Source: three-view drawing plus pictorial views. Frame: mm from the lowest corner of the part. A direction names the side the tool comes from. Give positions to 0.01 mm unless a question says otherwise; leave off trailing zeros. Write each loop counter-clockwise with the first axis right and the second up, starting at its lowest first coordinate (ties: lowest second). Pieces come first, ordered by that corner, then holes. Notation, with made-up numbers: (1, 17) -> (39, 17) arc R16 cw to (39, 47) -> close; hole circle Ø7 at (15.25, 10.5). An arc over 180 degrees is marked (long way). Answer in a Markdown table with one row per item. Add a question column.
Item 1: First-contact query: P1, Ø8, axis at x = 7.5, y = 37.5, coming from the +Z side; P2, Ø6, axis at x = 29.5, z = 18.5, coming from the +Y side; P3, Ø5, axis at x = 32.5, y = 7.5, coming from the -Z side (3 decimals); P4, Ø0.9, axis at x = 25, y = 12.5, coming from the +Z side. Flat tips, straight axial feed; report the tip coordinate or a pass-through.
Item 2: Material intervals for probe 1 along Y at (x, z) = (19, 29) (1 decimal); probe 2 along Z at (x, y) = (21, 35); probe 3 along Z at (x, y) = (20, 33), sorted ascending. Write a range as from..to.
Item 3: Draft query along Z for the marked faces 3, 4 and 5. Return one class per face: +Z half, -Z half, draft (parallel to the pull), parting line (faces both ways), or undercut.
Item 4: Section query C-C on z = 32. State how many separate pieces and enclosed holes the cut face has, plus the area to 3 significant figures.
Item 5: Access query for the marked faces 1 and 2. Directions: +Z, -Z, +X, -X, +Y, -Y. A direction counts if a zero-diameter tool reaches every point of the face in a straight line with its end or side. Return the directions, or none.
Item 6: Section query B-B on x = 19. Output: boundary loops of the cut face in (y, z) (1 decimal), plus the area to 3 significant figures.
Item 7: Section query A-A on y = 40. Output: boundary loops of the cut face in (x, z) (1 decimal).
Item 8: Section query D-D on z = 47. Output: boundary loops of the cut face in (x, y).
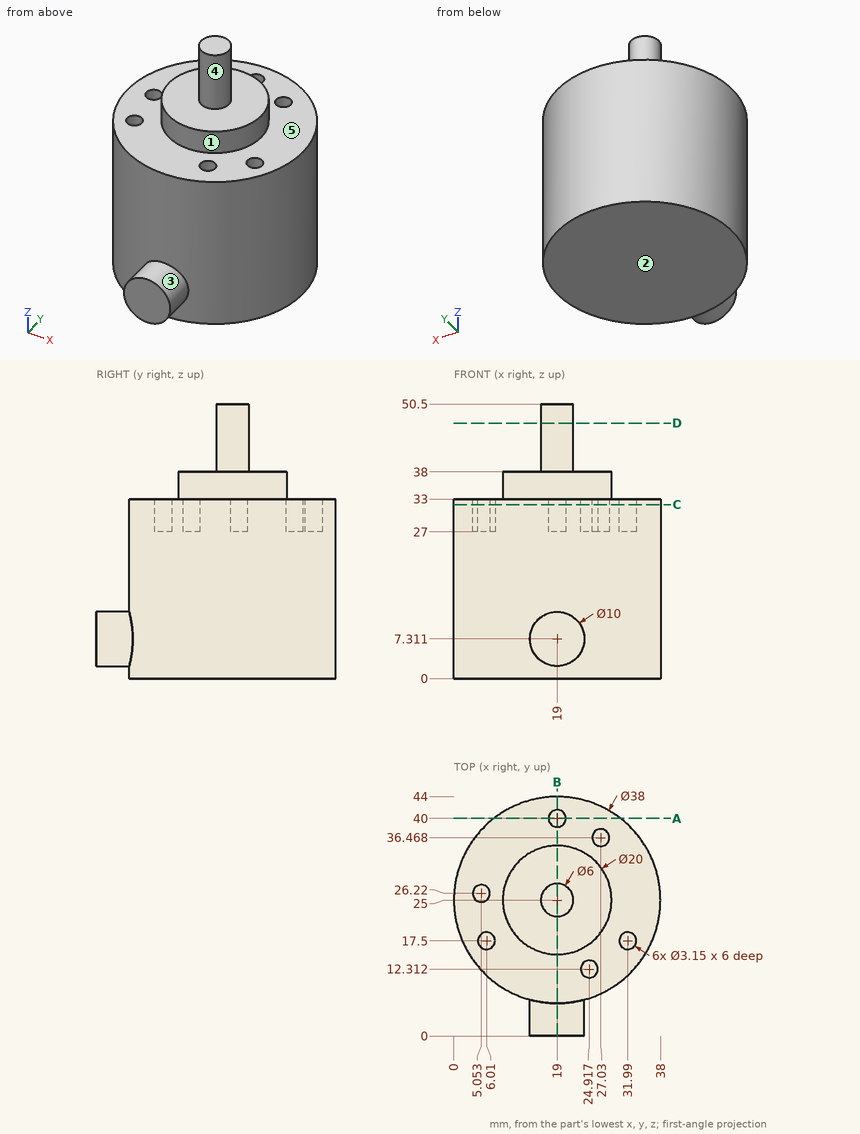
Findings below:
| question | item | result |
|---|---|---|
| 1 | P1 | stops at z = 33 |
| 1 | P2 | stops at y = 42.46 |
| 1 | P3 | passes through |
| 1 | P4 | stops at z = 27 |
| 2 | probe 1 | y = 6..38.4, 41.6..44 |
| 2 | probe 2 | z = 0..33 |
| 2 | probe 3 | z = 0..38 |
| 3 | face 3 | parting line |
| 3 | face 4 | draft |
| 3 | face 5 | +Z half |
| 4 | separate pieces | 1 |
| 4 | enclosed holes | 6 |
| 4 | area | 1,090 mm^2 |
| 5 | face 1 | +Z |
| 5 | face 2 | -Z, +X, -X, +Y, -Y |
| 6 | outline | (0, 2.3) -> (6, 2.3) -> (6, 0) -> (44, 0) -> (44, 33) -> (41.6, 33) -> (41.6, 27) -> (38.4, 27) -> (38.4, 33) -> (35, 33) -> (35, 38) -> (28, 38) -> (28, 50.5) -> (22, 50.5) -> (22, 38) -> (15, 38) -> (15, 33) -> (6, 33) -> (6, 12.3) -> (0, 12.3) -> close |
| 6 | area | 1,470 mm^2 |
| 7 | outline | (7.3, 0) -> (30.7, 0) -> (30.7, 33) -> (20.6, 33) -> (20.6, 27) -> (17.4, 27) -> (17.4, 33) -> (7.3, 33) -> close |
| 8 | outline | circle Ø6 at (19, 25) |
